from build123d import *

# Parameters (mm, degrees)
SKETCH1_R           = 20
SKETCH1_R_2         = 15
SKETCH1_R_3         = 40
SKETCH1_R_4         = 32
SKETCH1_R_5         = 21
SKETCH1_R_6         = 16
BOSS_EXTRUDE1_DEPTH = 17.5
BOSS_EXTRUDE2_START = -7.5
SKETCH1_5_R         = 15
BOSS_EXTRUDE2_DEPTH = 15


with BuildPart() as part:
    # Sketch1 → Boss-Extrude1 (new, symmetric)
    # profile 1 of 10: a face of its own
    with BuildSketch(Plane.XY):
        with Locations((-70, 0)):
            Circle(SKETCH1_R)
        with Locations((-70, 0)):
            Circle(SKETCH1_R_2, mode=Mode.SUBTRACT)
    # profile 2 of 10: a face of its own
    with BuildSketch(Plane.XY):
        with Locations((70, 0)):
            Circle(SKETCH1_R)
        with Locations((70, 0)):
            Circle(SKETCH1_R_2, mode=Mode.SUBTRACT)
    # profile 3 of 10: a face of its own
    with BuildSketch(Plane.XY):
        Circle(SKETCH1_R_3)
        Circle(SKETCH1_R_4, mode=Mode.SUBTRACT)
    # profile 4 of 10: a face of its own
    with BuildSketch(Plane.XY):
        Circle(SKETCH1_R_5)
        Circle(SKETCH1_R_6, mode=Mode.SUBTRACT)
    # profile 5 of 10: a face of its own
    with BuildSketch(Plane.XY):
        with BuildLine():
            ThreePointArc((20.406440309, -24.649080996), (22.627416998, -22.627416998), (24.649080996, -20.406440309))
            Line((24.649080996, -20.406440309), (16.8182588, -12.575618113))
            ThreePointArc((16.8182588, -12.575618113), (14.849242405, -14.849242405), (12.575618113, -16.8182588))
            Line((12.575618113, -16.8182588), (20.406440309, -24.649080996))
        make_face()
    # profile 6 of 10: a face of its own
    with BuildSketch(Plane.XY):
        with BuildLine():
            ThreePointArc((-3, -31.859064644), (0, -32), (3, -31.859064644))
            Line((3, -31.859064644), (3, -20.784609691))
            ThreePointArc((3, -20.784609691), (0, -21), (-3, -20.784609691))
            Line((-3, -20.784609691), (-3, -31.859064644))
        make_face()
    # profile 7 of 10: a face of its own
    with BuildSketch(Plane.XY):
        with BuildLine():
            Line((-16.8182588, -12.575618113), (-24.649080996, -20.406440309))
            ThreePointArc((-24.649080996, -20.406440309), (-22.627416998, -22.627416998), (-20.406440309, -24.649080996))
            Line((-20.406440309, -24.649080996), (-12.575618113, -16.8182588))
            ThreePointArc((-12.575618113, -16.8182588), (-14.849242405, -14.849242405), (-16.8182588, -12.575618113))
        make_face()
    # profile 8 of 10: a face of its own
    with BuildSketch(Plane.XY):
        with BuildLine():
            Line((-12.575618113, 16.8182588), (-20.406440309, 24.649080996))
            ThreePointArc((-20.406440309, 24.649080996), (-22.627416998, 22.627416998), (-24.649080996, 20.406440309))
            Line((-24.649080996, 20.406440309), (-16.8182588, 12.575618113))
            ThreePointArc((-16.8182588, 12.575618113), (-14.849242405, 14.849242405), (-12.575618113, 16.8182588))
        make_face()
    # profile 9 of 10: a face of its own
    with BuildSketch(Plane.XY):
        with BuildLine():
            Line((3, 20.784609691), (3, 31.859064644))
            ThreePointArc((3, 31.859064644), (0, 32), (-3, 31.859064644))
            Line((-3, 31.859064644), (-3, 20.784609691))
            ThreePointArc((-3, 20.784609691), (0, 21), (3, 20.784609691))
        make_face()
    # profile 10 of 10: a face of its own
    with BuildSketch(Plane.XY):
        with BuildLine():
            ThreePointArc((24.649080996, 20.406440309), (22.627416998, 22.627416998), (20.406440309, 24.649080996))
            Line((20.406440309, 24.649080996), (12.575618113, 16.8182588))
            ThreePointArc((12.575618113, 16.8182588), (14.849242405, 14.849242405), (16.8182588, 12.575618113))
            Line((16.8182588, 12.575618113), (24.649080996, 20.406440309))
        make_face()
    extrude(amount=BOSS_EXTRUDE1_DEPTH, both=True)

    # Sketch1<5> → Boss-Extrude2 (add)
    # profile 1 of 2: a face of its own
    with BuildSketch(Plane.XY.offset(BOSS_EXTRUDE2_START)):
        with BuildLine():
            ThreePointArc((-29.002885891, -59.651863383), (-22.168588856, -44.262528341), (-6.003756239, -39.546869801))
            ThreePointArc((-6.003756239, -39.546869801), (-40, 0), (-6.003756239, 39.546869801))
            ThreePointArc((-6.003756239, 39.546869801), (-22.168588856, 44.262528341), (-29.002885891, 59.651863383))
            ThreePointArc((-29.002885891, 59.651863383), (-46.639863286, 80.729435141), (-70.031947242, 66.302466954))
            Line((-70.031947242, 66.302466954), (-88.505015581, 7.587120556))
            ThreePointArc((-88.505015581, 7.587120556), (-66.133497163, 19.622694917), (-50, 0))
            ThreePointArc((-50, 0), (-66.133497163, -19.622694917), (-88.505015581, -7.587120556))
            Line((-88.505015581, -7.587120556), (-70.031947242, -66.302466954))
            ThreePointArc((-70.031947242, -66.302466954), (-46.639863286, -80.729435141), (-29.002885891, -59.651863383))
        make_face()
        with Locations((-50, -60)):
            Circle(SKETCH1_5_R, mode=Mode.SUBTRACT)
        with Locations((-50, 60)):
            Circle(SKETCH1_5_R, mode=Mode.SUBTRACT)
    # profile 2 of 2: a face of its own
    with BuildSketch(Plane.XY.offset(BOSS_EXTRUDE2_START)):
        with BuildLine():
            ThreePointArc((29.002885891, -59.651863383), (46.639863286, -80.729435141), (70.031947242, -66.302466954))
            Line((70.031947242, -66.302466954), (88.505015581, -7.587120556))
            ThreePointArc((88.505015581, -7.587120556), (50, 0), (88.505015581, 7.587120556))
            Line((88.505015581, 7.587120556), (70.031947242, 66.302466954))
            ThreePointArc((70.031947242, 66.302466954), (46.639863286, 80.729435141), (29.002885891, 59.651863383))
            ThreePointArc((29.002885891, 59.651863383), (22.168588856, 44.262528341), (6.003756239, 39.546869801))
            ThreePointArc((6.003756239, 39.546869801), (30.332740146, 26.075369129), (40, 0))
            ThreePointArc((40, 0), (30.332740146, -26.075369129), (6.003756239, -39.546869801))
            ThreePointArc((6.003756239, -39.546869801), (22.168588856, -44.262528341), (29.002885891, -59.651863383))
        make_face()
        with Locations((50, -60)):
            Circle(SKETCH1_5_R, mode=Mode.SUBTRACT)
        with Locations((50, 60)):
            Circle(SKETCH1_5_R, mode=Mode.SUBTRACT)
    extrude(amount=BOSS_EXTRUDE2_DEPTH)


solid = part.part
Can you work these out from the model? Positions are in its coordinate system, mm. A direction names the side the tool comes from. Round coordinates to 2 decimals unless told otherwise and drop trailing zeros. Write each loop counter-clockwise with the first axis right and the second up, starting at its lowest first coordinate (ties: lowest second). Pieces come first, ordered by that corner, then holes. Notation, with made-up numbers: M 75.25,32 L 118.25,32 A19 cw 118.25,40 Z; hole C 17.5,63.25 d6. An arc over 180 degrees is marked long. Use a Markdown table: item, result.
Item 1: We'd pull the mould along Y, two halves only. Please class faces 4 (the face through (3, -26, 0)), 5 (the face through (-67, 15, -17.5)), 6 (the face through (79.139, -37.356, -0.105)): released by +Y, released by -Y, zero draft, split by the parting line, or undercut.
Found:
| item | result |
|---|---|
| face 4 | undercut |
| face 5 | zero draft |
| face 6 | released by -Y |
Item 2: I want a section at A-A (x = 0). List the corners of the cut face in (y, z) for me, and give its area (3 significant figures).
Found:
| item | result |
|---|---|
| outline | M -40,-17.5 L -16,-17.5 L -16,17.5 L -40,17.5 Z; M 16,-17.5 L 40,-17.5 L 40,17.5 L 16,17.5 Z |
| area | 1,680 mm2 |
Item 3: For pin 1 Ø2 at (x, y) = (45, 36.5) entering from +Z; pin 2 Ø3 at (x, z) = (-25, 6.5) entering from -Y; pin 3 Ø10 at (x, z) = (-68.5, 14) entering from +Y, each with a flat end and sliding along its axis, tell me the tip position at first contact or that it passes through.
Found:
| item | result |
|---|---|
| pin 1 | stops at z = 7.5 |
| pin 2 | stops at y = -49.63 |
| pin 3 | stops at y = 20 |
Item 4: If I drill on line 1 along Y through (x, z) = (-50, -4); line 2 along Y through (x, z) = (0.5, 9); line 3 along Y through (x, z) = (5.5, 6), over which ranges is the centre line in solid material (lowest first)? Write a range as [from, to].
Found:
| item | result |
|---|---|
| line 1 | y = [-81, -75], [-45, 45], [75, 81] |
| line 2 | y = [-40, -15.99], [15.99, 40] |
| line 3 | y = [-39.62, -31.52], [-20.27, -15.02], [15.02, 20.27], [31.52, 39.62] |
Item 5: I want a section at C-C (y = 63). List the corners of the cut face in (x, z) for me, and give its area (3 significant figures).
Found:
| item | result |
|---|---|
| outline | M -71.07,-7.5 L -64.7,-7.5 L -64.7,7.5 L -71.07,7.5 Z; M -35.3,-7.5 L -29.22,-7.5 L -29.22,7.5 L -35.3,7.5 Z; M 29.22,-7.5 L 35.3,-7.5 L 35.3,7.5 L 29.22,7.5 Z; M 64.7,-7.5 L 71.07,-7.5 L 71.07,7.5 L 64.7,7.5 Z |
| area | 374 mm2 |
Item 6: Which directions (+Z, -Z, +X, -X, +Y, -Y) give clear straight access to the entire face, cutting with the end or side of a thin tool? Please do faces 1 (the face through (47, 1, 7.5)), 2 (the face through (-16.44, 20.68, -0.25)), 3 (the face through (-79.139, 37.356, -0.105)).
Found:
| item | result |
|---|---|
| face 1 | +Z |
| face 2 | +Z, -Z |
| face 3 | +Z, -Z, -X, +Y |
Item 7: I want a section at B-B (z = 14.5). State how many separate pieces and enclosed holes the cut face has, and give its area (3 significant figures).
Found:
| item | result |
|---|---|
| separate pieces | 3 |
| enclosed holes | 9 |
| area | 3,890 mm2 |
